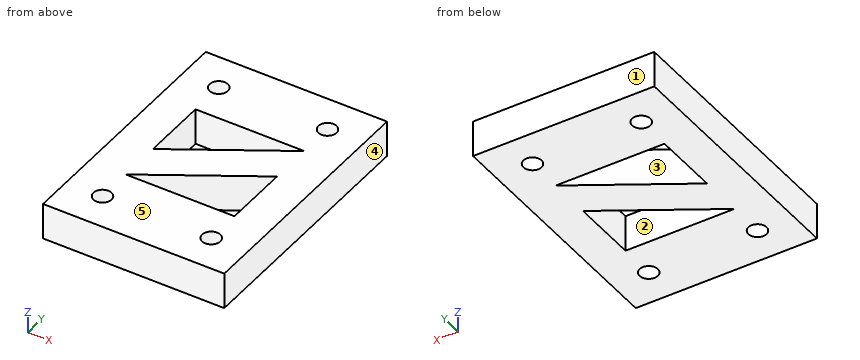
```python
from build123d import *

# Parameters (mm, degrees)
SKETCH1_W          = 50
SKETCH1_H          = 70
BASE_FLANGE1_DEPTH = 10
CUT_EXTRUDE1_REACH = 88.603
SKETCH6_R          = 2.5


# Sheet-metal steps are written as plain solids
with BuildPart() as part:
    # Sketch1 → Base-Flange1 (new body)
    with BuildSketch(Plane.XY):
        with Locations((25, 35)):
            Rectangle(SKETCH1_W, SKETCH1_H)
    extrude(amount=-BASE_FLANGE1_DEPTH)

    # Sketch6 → Cut-Extrude1 (cut, up to next)
    with BuildSketch(Plane.XY, mode=Mode.PRIVATE) as cut_extrude1_sk1:
        with Locations((40, 60)):
            Circle(SKETCH6_R)
    cut_extrude1_tool1 = extrude(cut_extrude1_sk1.sketch, amount=-CUT_EXTRUDE1_REACH, mode=Mode.PRIVATE) & part.part
    # Sketch6 → Cut-Extrude1 (cut, up to next)
    with BuildSketch(Plane.XY, mode=Mode.PRIVATE) as cut_extrude1_sk2:
        with Locations((10, 10)):
            Circle(SKETCH6_R)
    cut_extrude1_tool2 = extrude(cut_extrude1_sk2.sketch, amount=-CUT_EXTRUDE1_REACH, mode=Mode.PRIVATE) & part.part
    # Sketch6 → Cut-Extrude1 (cut, up to next)
    with BuildSketch(Plane.XY, mode=Mode.PRIVATE) as cut_extrude1_sk3:
        with Locations(Location((10, 60, 0), (0, 0, 180))):
            Circle(SKETCH6_R)
    cut_extrude1_tool3 = extrude(cut_extrude1_sk3.sketch, amount=-CUT_EXTRUDE1_REACH, mode=Mode.PRIVATE) & part.part
    # Sketch6 → Cut-Extrude1 (cut, up to next)
    with BuildSketch(Plane.XY, mode=Mode.PRIVATE) as cut_extrude1_sk4:
        with Locations(Location((40, 10, 0), (0, 0, 180))):
            Circle(SKETCH6_R)
    cut_extrude1_tool4 = extrude(cut_extrude1_sk4.sketch, amount=-CUT_EXTRUDE1_REACH, mode=Mode.PRIVATE) & part.part
    # Sketch6 → Cut-Extrude1 (cut, up to next)
    with BuildSketch(Plane.XY, mode=Mode.PRIVATE) as cut_extrude1_sk5:
        Polygon((40, 38.288353904), (40, 20), (10, 20), align=None)
    cut_extrude1_tool5 = extrude(cut_extrude1_sk5.sketch, amount=-CUT_EXTRUDE1_REACH, mode=Mode.PRIVATE) & part.part
    # Sketch6 → Cut-Extrude1 (cut, up to next)
    with BuildSketch(Plane.XY, mode=Mode.PRIVATE) as cut_extrude1_sk6:
        Polygon((40, 50), (10, 31.711646096), (10, 50), align=None)
    cut_extrude1_tool6 = extrude(cut_extrude1_sk6.sketch, amount=-CUT_EXTRUDE1_REACH, mode=Mode.PRIVATE) & part.part
    add(cut_extrude1_tool1.solids().sort_by_distance((40, 60, 0))[0], mode=Mode.SUBTRACT)
    add(cut_extrude1_tool2.solids().sort_by_distance((10, 10, 0))[0], mode=Mode.SUBTRACT)
    add(cut_extrude1_tool3.solids().sort_by_distance((10, 60, 0))[0], mode=Mode.SUBTRACT)
    add(cut_extrude1_tool4.solids().sort_by_distance((40, 10, 0))[0], mode=Mode.SUBTRACT)
    add(cut_extrude1_tool5.solids().sort_by_distance((30, 26.096118, 0))[0], mode=Mode.SUBTRACT)
    add(cut_extrude1_tool6.solids().sort_by_distance((20, 43.903882, 0))[0], mode=Mode.SUBTRACT)


solid = part.part
```
Check sheet for the modelled part. Datum: model origin and axes. Units: mm. Face numbers are marked on the shaded views. A direction names the side the tool comes from. Round coordinates to 2 decimals unless told otherwise and drop trailing zeros. Order: outer loops, then holes, each group sorted by start corner. A loop starts at its lowest first (then second) coordinate and runs counter-clockwise, first axis right, second up. Notation, with made-up numbers: M 4,27 L 9,27 A22 ccw 9,34 Z; hole C 50,32.5 d11. An arc over 180 degrees is marked long. Answer in a Markdown table with one row per item.
(1) Section check D-D on x = 38.5. Record the boundary of the cut face in (y, z).
Findings:
| item | result |
|---|---|
| outline | M 0,-10 L 8,-10 L 8,0 L 0,0 Z; M 12,-10 L 20,-10 L 20,0 L 12,0 Z; M 37.37,-10 L 49.09,-10 L 49.09,0 L 37.37,0 Z; M 50,-10 L 58,-10 L 58,0 L 50,0 Z; M 62,-10 L 70,-10 L 70,0 L 62,0 Z |
(2) Section check B-B on z = -8.75. Record the boundary of the cut face in (x, y), plus the area to 3 significant figures.
Findings:
| item | result |
|---|---|
| outline | M 0,0 L 50,0 L 50,70 L 0,70 Z; hole C 10,10 d5; hole C 10,60 d5; hole M 10,20 L 40,20 L 40,38.29 Z; hole M 10,31.71 L 40,50 L 10,50 Z; hole C 40,10 d5; hole C 40,60 d5 |
| area | 2,870 mm^2 |
(3) Draft check along X on the marked faces 3, 4 and 5. Enter one of: +X half, -X half, draft (parallel to the pull), parting line (faces both ways), or undercut.
Findings:
| item | result |
|---|---|
| face 3 | undercut |
| face 4 | +X half |
| face 5 | draft |
(4) Section check A-A on y = 61.5. Record the boundary of the cut face in (x, z), plus the area to 3 significant figures.
Findings:
| item | result |
|---|---|
| outline | M 0,-10 L 8,-10 L 8,0 L 0,0 Z; M 12,-10 L 38,-10 L 38,0 L 12,0 Z; M 42,-10 L 50,-10 L 50,0 L 42,0 Z |
| area | 420 mm^2 |
(5) Section check C-C on x = 20.5. Record the boundary of the cut face in (y, z), plus the area to 3 significant figures.
Findings:
| item | result |
|---|---|
| outline | M 0,-10 L 20,-10 L 20,0 L 0,0 Z; M 26.4,-10 L 38.11,-10 L 38.11,0 L 26.4,0 Z; M 50,-10 L 70,-10 L 70,0 L 50,0 Z |
| area | 517 mm^2 |
(6) Set-up check for the marked faces 1 and 2: record each of +Z, -Z, +X, -X, +Y, -Y from which the full face is reachable in a straight line by a thin tool's end or side.
Findings:
| item | result |
|---|---|
| face 1 | +Z, -Z, +X, -X, +Y |
| face 2 | +Z, -Z |
(7) Material ranges on line 1 along X through (y, z) = (33, -7.5); line 2 along X through (y, z) = (35, -6.75); line 3 along Y through (x, z) = (39.5, -3.5), recorded low to high. Write a range as from..to.
Findings:
| item | result |
|---|---|
| line 1 | x = 0..10, 12.11..31.33, 40..50 |
| line 2 | x = 0..10, 15.39..34.61, 40..50 |
| line 3 | y = 0..7.55, 12.45..20, 37.98..49.7, 50..57.55, 62.45..70 |
